Read the model definition and answer for the solid it produces. Units are mm, in the model's axes. A direction names the side the tool comes from. Coordinates: 2 decimals unless noted, no trailing zeros. Loops run counter-clockwise (first coordinate to the right, second up) from the corner with the lowest first, then second, coordinate; pieces in that order, holes last. Notation, with made-up numbers: (-20, 76) - (-12, 76) arc R17 ccw to (-12, 106) - close; hole circle Ø6 at (46.25, 45.5). An arc over 180 degrees is marked (long way). One line per item, written item: value. Start each with the question number.
Autodesk Inventor part; units mm, degrees
ref_plane "YZ Plane" through (0, 0, 0) normal (1, 0, 0) x (0, 1, 0)
ref_plane "XZ Plane" through (0, 0, 0) normal (0, 1, 0) x (-1, 0, 0)
ref_plane "XY Plane" through (0, 0, 0) normal (0, 0, 1) x (1, 0, 0)
sketch "Sketch1" plane through (0, 0, 0) normal (0, 0, 1) x (1, 0, 0)
  line L0 (2, 0) -> (51.18, 0)
  line L1 (53.18, 2) -> (53.18, 34.924)
  line L2 (51.18, 36.924) -> (2, 36.924)
  line L3 (0, 34.924) -> (0, 2)
  arc A0 (2, 36.924) -> (0, 34.924) centre (2, 34.924) ccw
  arc A1 (0, 2) -> (2, 0) centre (2, 2) ccw
  arc A2 (51.18, 0) -> (53.18, 2) centre (51.18, 2) ccw
  arc A3 (53.18, 34.924) -> (51.18, 36.924) centre (51.18, 34.924) ccw
  point P0 (0, 0)
  point P1 (53.18, 36.924)
  point P2 (53.18, 0)
  point P3 (0, 36.924)
  dimension "d0" = 36.924
  dimension "d1" = 53.18
  dimension "d2" = 2
extrude "Extrusion1" add sketch "Sketch1" along normal blind 2
sketch "Sketch2" plane through (0, 0, 2) normal (0, 0, 1) x (1, 0, 0)
  point P0 (0, 0)
sketch "Sketch3" plane through (0, 0, 2) normal (0, 0, 1) x (1, 0, 0)
  line L0 (3.9641, 27.5862) -> (4.2577, 27.5862)
  line L1 (4.2577, 27.5862) -> (4.2577, 27.8798)
  line L2 (4.2577, 27.8798) -> (3.9641, 27.8798)
  line L3 (3.9641, 27.8798) -> (3.9641, 27.5862)
  line L4 (3.9793, 10.8373) -> (4.2425, 10.8373)
  line L5 (4.2425, 10.8373) -> (4.2425, 11.1006)
  line L6 (4.2425, 11.1006) -> (3.9793, 11.1006)
  line L7 (3.9793, 11.1006) -> (3.9793, 10.8373)
  line L8 (2.5409, 9.399) -> (5.6809, 9.399)
  line L9 (5.6809, 9.399) -> (5.6809, 29.303)
  line L10 (5.6809, 29.303) -> (2.5409, 29.303)
  line L11 (2.5409, 29.303) -> (2.5409, 9.399)
  line L12 (36.7302, 32.8328) -> (36.7302, 32.5392)
  line L13 (36.7302, 32.5392) -> (37.0238, 32.5392)
  line L14 (37.0238, 32.5392) -> (37.0238, 32.8328)
  line L15 (37.0238, 32.8328) -> (36.7302, 32.8328)
  line L16 (39.2702, 32.8328) -> (39.2702, 32.5392)
  line L17 (39.2702, 32.5392) -> (39.5638, 32.5392)
  line L18 (39.5638, 32.5392) -> (39.5638, 32.8328)
  line L19 (39.5638, 32.8328) -> (39.2702, 32.8328)
  line L20 (35.307, 34.256) -> (40.987, 34.256)
  line L21 (40.987, 34.256) -> (40.987, 31.116)
  line L22 (40.987, 31.116) -> (35.307, 31.116)
  line L23 (35.307, 31.116) -> (35.307, 34.256)
  arc A0 (51.18, 0) -> (53.18, 2) centre (51.18, 2) ccw
  line L24 (53.18, 2) -> (53.18, 34.924)
  arc A1 (53.18, 34.924) -> (51.18, 36.924) centre (51.18, 34.924) ccw
  line L25 (51.18, 36.924) -> (2, 36.924)
  arc A2 (2, 36.924) -> (0, 34.924) centre (2, 34.924) ccw
  line L26 (0, 34.924) -> (0, 2)
  arc A3 (0, 2) -> (2, 0) centre (2, 2) ccw
  line L27 (2, 0) -> (51.18, 0)
  line L28 (49.341, 10.949) -> (27.8799, 10.949) construction
  line L29 (27.8799, 10.949) -> (27.8799, 21.149) construction
  line L30 (27.8799, 21.149) -> (49.341, 21.149) construction
  line L31 (49.341, 21.149) -> (49.341, 10.949) construction
  line L32 (49.741, 10.549) -> (27.4799, 10.549)
  line L33 (27.4799, 10.549) -> (27.4799, 21.549)
  line L34 (27.4799, 21.549) -> (49.741, 21.549) construction
  line L35 (49.741, 21.549) -> (49.741, 10.549)
  line L36 (49.741, 21.549) -> (27.4799, 21.549) construction
  line L37 (27.4799, 21.549) -> (27.4799, 29.0699)
  line L38 (27.4799, 29.0699) -> (49.741, 29.0699) construction
  line L39 (49.741, 29.0699) -> (49.741, 21.549)
  line L40 (27.4799, 29.0699) -> (49.741, 29.0699)
  line L41 (49.741, 29.0699) -> (49.741, 29.4699)
  line L42 (49.741, 29.4699) -> (27.4799, 29.4699)
  line L43 (27.4799, 29.4699) -> (27.4799, 29.0699)
  line L44 (37.1719, 9.3139) -> (45.4719, 9.3139)
  line L45 (45.4719, 9.3139) -> (45.4719, 2.7139)
  line L46 (45.4719, 2.7139) -> (37.1719, 2.7139)
  line L47 (37.1719, 2.7139) -> (37.1719, 9.3139)
  point P0 (0, 0)
  point P1 (3.9793, 10.969)
  point P2 (4.1109, 11.1006)
  point P3 (4.1109, 9.399)
  point P4 (4.1109, 29.303)
  point P5 (3.9641, 27.733)
  point P6 (36.877, 32.8328)
  point P7 (39.417, 32.8328)
  point P8 (39.5638, 32.686)
  point P9 (40.987, 32.686)
  point P10 (27.8799, 11.076)
  point P11 (27.883, 21.5699)
  point P12 (49.304, 29.0699)
  point P13 (49.304, 21.5699)
  point P14 (27.883, 29.0699)
  point P15 (37.5719, 8.9139)
  point P16 (45.0719, 3.1139)
  dimension "d5" = 1.57
  dimension "d6" = 1.57
  dimension "d7" = 1.57
  dimension "d8" = 1.57
  dimension "d9" = 1.57
  dimension "d10" = 1.57
  dimension "d13" = 0.4
  dimension "d14" = 0.4
  dimension "d15" = 0.4
  dimension "d16" = 0.4
  dimension "d17" = 0.4
  dimension "d18" = 0.4
  dimension "d19" = 0.4
  dimension "d20" = 0.4
  dimension "d21" = 0.4
extrude "Extrusion2" cut sketch "Sketch3" against normal through all contours L3 L2 L1 L0 | L7 L6 L5 L4 | L11 L10 L9 L8 | L15 L14 L13 L12 | L19 L18 L17 L16 | L20 L21 L22 L23 | L32 L33 L37 L40 L39 L35 | L40 L43 L42 L41 | L44 L45 L46 L47
sketch "Sketch4" plane through (0, 0, 0) normal (0, 0, -1) x (-1, 0, 0)
  arc A0 (-2, 0) -> (0, 2) centre (-2, 2) ccw
  line L0 (0, 2) -> (0, 34.924)
  line L1 (-51.18, 0) -> (-2, 0)
  arc A1 (-53.18, 2) -> (-51.18, 0) centre (-51.18, 2) ccw
  line L2 (-53.18, 34.924) -> (-53.18, 2)
  arc A2 (-51.18, 36.924) -> (-53.18, 34.924) centre (-51.18, 34.924) ccw
  line L3 (-2, 36.924) -> (-51.18, 36.924)
  arc A3 (0, 34.924) -> (-2, 36.924) centre (-2, 34.924) ccw
  point P0 (0, 0)
extrude "Extrusion3" add sketch "Sketch4" along normal blind 15 separate body
shell "Shell1" thickness 1.6 removed faces 3 at (12.9473, 16.417, 0) at (34.7867, 12.308, 0) at (34.7867, 12.308, -15) bodies 2
combine bodies "Combine1" operation type add bodies to combine 1 2
properties part number "Frame_Lid"
1) Section A-A, the plane y = 10 is taken. Determine the outline of the cut face in (x, z), and give its area (3 significant figures).
2) Section D-D, the plane z = 1 is taken. Determine the outline of the cut face in (x, y).
3) Section C-C, the plane x = 3.5 is taken. Determine the outline of the cut face in (y, z), and give its area (3 significant figures).
4) Determine the mould class of faces 1 (the flat face through (26, 0, -7)), 2 (the flat face through (29, 1, -15)), 3 (the flat face through (41, 2.714, 1)) for opening direction Y: released by +Y, released by -Y, zero draft, split by the parting line, or undercut.
5) A flat-ended cylindrical pin translates along its axis: P1, Ø17, axis at x = 33.5, y = 12, coming from the -Z side. Find the tip coordinate at first contact, or state that the pin passes through.
6) For faces 4 (the flat face through (27, 1.6, -7)), 5 (the flat face through (53.18, 18, -7)), 6 (the flat face through (4, 9.399, 1)), determine the directions among +Z, -Z, +X, -X, +Y, -Y from which every point of the face is accessible in a straight line to the end or side of a thin tool.
7) Straight lines are drawn through the part: L1, parallel to X at y = 5.5, z = -13.5; L2, parallel to Y at x = 37, z = -1.5; L3, parallel to Z at x = 14.5, y = 11.5. For each, find the intervals that lie inside material, in ascending order.
8) Section B-B, the plane y = 25.5 is taken. Determine the outline of the cut face in (x, z).
Answer below:
1. outline: (0, -15) - (1.6, -15) - (1.6, 0) - (2.54, 0) - (2.54, 2) - (0, 2) - close; (5.68, 0) - (51.58, 0) - (51.58, -15) - (53.18, -15) - (53.18, 2) - (5.68, 2) - close
1. area: 148 mm2
2. outline: (0, 2) arc R2 ccw to (2, 0) - (51.18, 0) arc R2 ccw to (53.18, 2) - (53.18, 34.92) arc R2 ccw to (51.18, 36.92) - (2, 36.92) arc R2 ccw to (0, 34.92) - close; hole (2.54, 9.4) - (5.68, 9.4) - (5.68, 29.3) - (2.54, 29.3) - close; hole (27.48, 10.55) - (49.74, 10.55) - (49.74, 29.47) - (27.48, 29.47) - close; hole (35.31, 31.12) - (40.99, 31.12) - (40.99, 34.26) - (35.31, 34.26) - close; hole (37.17, 2.71) - (45.47, 2.71) - (45.47, 9.31) - (37.17, 9.31) - close
3. outline: (0, -15) - (1.6, -15) - (1.6, 0) - (9.4, 0) - (9.4, 2) - (0, 2) - close; (29.3, 0) - (35.32, 0) - (35.32, -15) - (36.92, -15) - (36.92, 2) - (29.3, 2) - close
3. area: 82.0 mm2
4. face 1: released by -Y
4. face 2: zero draft
4. face 3: undercut
5. P1: z = 0
6. face 4: -Z
6. face 5: +Z, -Z, +X, +Y, -Y
6. face 6: +Z, -Z
7. L1: 0 to 1.6, 51.58 to 53.18
7. L2: 0 to 1.6, 35.32 to 36.92
7. L3: 0 to 2
8. outline: (0, -15) - (1.6, -15) - (1.6, 0) - (2.54, 0) - (2.54, 2) - (0, 2) - close; (5.68, 0) - (27.48, 0) - (27.48, 2) - (5.68, 2) - close; (49.74, 0) - (51.58, 0) - (51.58, -15) - (53.18, -15) - (53.18, 2) - (49.74, 2) - close
